Verification items for the finished model (mm, model axes). Face numbers are marked on the shaded views. A direction names the side the tool comes from. Give positions to 0.01 mm unless a question says otherwise; leave off trailing zeros. Order: outer loops, then holes, each group sorted by start corner. A loop starts at its lowest first (then second) coordinate and runs counter-clockwise, first axis right, second up.
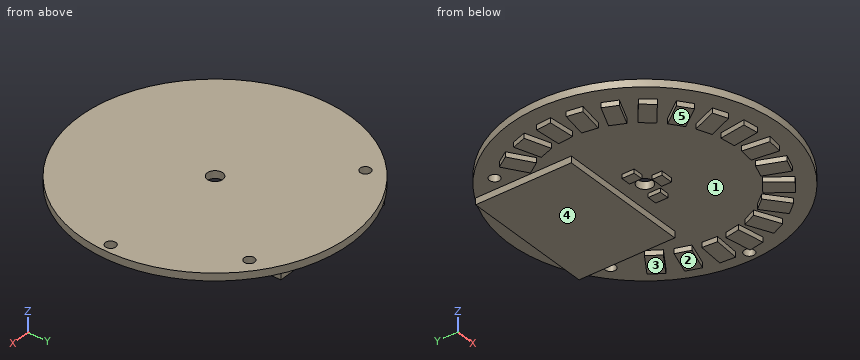
from build123d import *

# Parameters (mm, degrees)
SKETCH_1_R           = 27.25
SKETCH_1_R_2         = 1.05
SKETCH_1_R_3         = 1.55
EXTRUDE_1_DEPTH      = 1.5
SKETCH_2_W           = 26.7
SKETCH_2_H           = 19.2
EXTRUDE_2_DEPTH      = 1.3
BOSS_EXTRUDE1_DEPTH  = 1
CIRPATTERN1_COUNT    = 9
CIRPATTERN1_ANGLE    = 116
SKETCH2_W            = 2.46
SKETCH2_H            = 1.96
SKETCH2_W_2          = 1.96
SKETCH2_H_2          = 2.46
BOSS_EXTRUDE2_DEPTH  = 0.8
MIRROR1_COPY_1_DEPTH = 1
MIRROR1_COPY_2_DEPTH = 1
MIRROR1_COPY_3_DEPTH = 1
MIRROR1_COPY_4_DEPTH = 1
MIRROR1_COPY_5_DEPTH = 1
MIRROR1_COPY_6_DEPTH = 1
MIRROR1_COPY_7_DEPTH = 1
MIRROR1_COPY_8_DEPTH = 1


with BuildPart() as part:
    # Эскиз1 → Бобышка-Вытянуть1 (new body)
    with BuildSketch(Plane.XY):
        Circle(SKETCH_1_R)
        with Locations((-15.9, 17.8)):
            Circle(SKETCH_1_R_2, mode=Mode.SUBTRACT)
        with Locations((15.25, 18.75)):
            Circle(SKETCH_1_R_2, mode=Mode.SUBTRACT)
        with Locations((25.35, -1.23)):
            Circle(SKETCH_1_R_2, mode=Mode.SUBTRACT)
        Circle(SKETCH_1_R_3, mode=Mode.SUBTRACT)
    extrude(amount=EXTRUDE_1_DEPTH)

    # Эскиз2 → Бобышка-Вытянуть2 (add)
    with BuildSketch(Plane.XY):
        with Locations((0, 14)):
            Rectangle(SKETCH_2_W, SKETCH_2_H)
    extrude(amount=-EXTRUDE_2_DEPTH)

    # Sketch1 → Boss-Extrude1 (add)
    with BuildSketch(Plane(origin=(0, 0, 0), x_dir=(-1, 0, 0), z_dir=(0, 0, -1))):
        Polygon((19.047763091, 14.406246778), (20.703574047, 11.904589312), (16.367367772, 9.034516988), (14.711556816, 11.536174454), align=None)
    boss_extrude1 = extrude(amount=BOSS_EXTRUDE1_DEPTH)

    # CirPattern1: Boss-Extrude1 ×9 about axis
    cirpattern1_axis = Axis((0, 0, 0), (0, 0, 1))
    for i in range(1, CIRPATTERN1_COUNT):
        add(boss_extrude1.rotate(cirpattern1_axis, i * CIRPATTERN1_ANGLE / (CIRPATTERN1_COUNT - 1)))

    # Sketch2 → Boss-Extrude2 (add)
    with BuildSketch(Plane(origin=(0, 0, 0), x_dir=(-1, 0, 0), z_dir=(0, 0, -1))):
        with Locations((0, -3.38)):
            Rectangle(SKETCH2_W, SKETCH2_H)
        with Locations((-3.38, 0)):
            Rectangle(SKETCH2_W_2, SKETCH2_H_2)
        with Locations((3.38, 0)):
            Rectangle(SKETCH2_W_2, SKETCH2_H_2)
    extrude(amount=BOSS_EXTRUDE2_DEPTH)

    # Mirror1: Boss-Extrude1 across plane
    add(boss_extrude1.mirror(Plane(origin=(0, 0, 0), x_dir=(0, 0, 1), z_dir=(1, 0, 0))))

    # Mirror1 copy 1 sketch → Mirror1 copy 1 (add)
    with BuildSketch(Plane(origin=(0, 0, 0), x_dir=(0.9681476403781076, -0.25038000405444194, 0), z_dir=(0, 0, -1))):
        Polygon((19.047763091, -14.406246778), (20.703574047, -11.904589312), (16.367367772, -9.034516988), (14.711556816, -11.536174454), align=None)
    extrude(amount=MIRROR1_COPY_1_DEPTH)

    # Mirror1 copy 2 sketch → Mirror1 copy 2 (add)
    with BuildSketch(Plane(origin=(0, 0, 0), x_dir=(0.8746197071393953, -0.484809620246338, 0), z_dir=(0, 0, -1))):
        Polygon((19.047763091, -14.406246778), (20.703574047, -11.904589312), (16.367367772, -9.034516988), (14.711556816, -11.536174454), align=None)
    extrude(amount=MIRROR1_COPY_2_DEPTH)

    # Mirror1 copy 3 sketch → Mirror1 copy 3 (add)
    with BuildSketch(Plane(origin=(0, 0, 0), x_dir=(0.7253743710122864, -0.6883545756937552, 0), z_dir=(0, 0, -1))):
        Polygon((19.047763091, -14.406246778), (20.703574047, -11.904589312), (16.367367772, -9.034516988), (14.711556816, -11.536174454), align=None)
    extrude(amount=MIRROR1_COPY_3_DEPTH)

    # Mirror1 copy 4 sketch → Mirror1 copy 4 (add)
    with BuildSketch(Plane(origin=(0, 0, 0), x_dir=(0.529919264233203, -0.8480480961564272, 0), z_dir=(0, 0, -1))):
        Polygon((19.047763091, -14.406246778), (20.703574047, -11.904589312), (16.367367772, -9.034516988), (14.711556816, -11.536174454), align=None)
    extrude(amount=MIRROR1_COPY_4_DEPTH)

    # Mirror1 copy 5 sketch → Mirror1 copy 5 (add)
    with BuildSketch(Plane(origin=(0, 0, 0), x_dir=(0.3007057995042705, -0.9537169507482277, 0), z_dir=(0, 0, -1))):
        Polygon((19.047763091, -14.406246778), (20.703574047, -11.904589312), (16.367367772, -9.034516988), (14.711556816, -11.536174454), align=None)
    extrude(amount=MIRROR1_COPY_5_DEPTH)

    # Mirror1 copy 6 sketch → Mirror1 copy 6 (add)
    with BuildSketch(Plane(origin=(0, 0, 0), x_dir=(0.05233595624294042, -0.998629534754574, 0), z_dir=(0, 0, -1))):
        Polygon((19.047763091, -14.406246778), (20.703574047, -11.904589312), (16.367367772, -9.034516988), (14.711556816, -11.536174454), align=None)
    extrude(amount=MIRROR1_COPY_6_DEPTH)

    # Mirror1 copy 7 sketch → Mirror1 copy 7 (add)
    with BuildSketch(Plane(origin=(0, 0, 0), x_dir=(-0.199367934417201, -0.9799247046208288, 0), z_dir=(0, 0, -1))):
        Polygon((19.047763091, -14.406246778), (20.703574047, -11.904589312), (16.367367772, -9.034516988), (14.711556816, -11.536174454), align=None)
    extrude(amount=MIRROR1_COPY_7_DEPTH)

    # Mirror1 copy 8 sketch → Mirror1 copy 8 (add)
    with BuildSketch(Plane(origin=(0, 0, 0), x_dir=(-0.4383711467890815, -0.898794046299165, 0), z_dir=(0, 0, -1))):
        Polygon((19.047763091, -14.406246778), (20.703574047, -11.904589312), (16.367367772, -9.034516988), (14.711556816, -11.536174454), align=None)
    extrude(amount=MIRROR1_COPY_8_DEPTH)


solid = part.part
(1) Set-up check for the marked faces 3, 4 and 5: record each of +Z, -Z, +X, -X, +Y, -Y from which the full face is reachable in a straight line by a thin tool's end or side.
Solved:
face 3: -Z, +X, +Y, -Y
face 4: -Z, +X, -X, +Y, -Y
face 5: -Z, +X, -X, -Y
(2) Section check C-C, the plane x = 6.5. Enter the section's corners in (y, z).
Solved:
outline: (-26.46, 0) - (-20.09, 0) - (-20.09, -1) - (-17.47, -1) - (-17.47, 0) - (4.4, 0) - (4.4, -1.3) - (23.6, -1.3) - (23.6, 0) - (26.46, 0) - (26.46, 1.5) - (-26.46, 1.5) - close
(3) Section check A-A, the plane x = 25.35. Enter the section's corners in (y, z), then the cut area to 3 significant figures.
Solved:
outline: (-10, 0) - (-2.28, 0) - (-2.28, 1.5) - (-10, 1.5) - close; (-0.18, 0) - (10, 0) - (10, 1.5) - (-0.18, 1.5) - close
area: 26.8 mm2
(4) Scan lines: line 1 (Y direction, x = 0, z = 0.6); line 2 (Z direction, x = -15.5, y = 6); line 3 (Z direction, x = -21, y = 3). Record each from-to range of solid material in increasing order.
Solved:
line 1: y = -27.25 to -1.55, 1.55 to 27.25
line 2: z = 0 to 1.5
line 3: z = -1 to 1.5
(5) Section check B-B, the plane z = 0.95. Enter the section's corners in (x, y).
Solved:
outline: circle Ø54.5 at (0, 0); hole circle Ø2.1 at (-15.9, 17.8); hole circle Ø3.1 at (0, 0); hole circle Ø2.1 at (15.25, 18.75); hole circle Ø2.1 at (25.35, -1.23)
(6) Release check for a two-part mould opening along Y. For the marked faces 1 and 2 record: pulls with the +Y half, pulls with the -Y half, needs draft (parallel to the pull), parting line crosses it, or undercut.
Solved:
face 1: undercut
face 2: needs draft
(7) Go/stop test with flat-tipped pins: pin 1 (5.5 mm diameter, centred on x = 19.5, y = -8, fed in from -Z); pin 2 (2.5 mm diameter, centred on x = 15.25, y = 18.75, fed in from -Z); pin 3 (0.9 mm diameter, centred on y = 0, z = -0.5, fed in from +X); pin 4 (3.5 mm diameter, centred on x = 0, y = 0, fed in from +Z). Record where each tip stops, or that it passes through.
Solved:
pin 1: stops at z = -1
pin 2: stops at z = 0
pin 3: stops at x = 23.88
pin 4: stops at z = 1.5
